Geometry check sheet. Reference: the model listing, model coordinates, mm. Face numbers are marked on the shaded views. A direction names the side the tool comes from. Coordinates: 2 decimals unless noted, no trailing zeros. Loops run counter-clockwise (first coordinate to the right, second up) from the corner with the lowest first, then second, coordinate; pieces in that order, holes last. Notation, with made-up numbers: (-3, 83.25) - (13, 83.25) arc R21 ccw to (13, 122.25) - close; hole circle Ø1 at (85, -5.5). An arc over 180 degrees is marked (long way). Write each question's results on one line, items separated by ' | '. Start each with the question number.
(1) Sectioned sample at B-B (z = 9.1). Enter the section's corners in (x, y), plus the area to 3 significant figures.
(2) Sectioned sample at A-A (y = 128.35). Enter the section's corners in (x, z), plus the area to 3 significant figures.
(3) Sectioned sample at D-D (x = -32.5). Enter the section's corners in (y, z), plus the area to 3 significant figures.
(4) Material ranges on probe 1 along Z at (x, y) = (-34, 166.05); probe 2 along Y at (x, z) = (-12, 9); probe 3 along Z at (x, y) = (-34, 167.8), recorded low to high.
(5) Access from +Z, -Z, +X, -X, +Y, -Y to the whole of each face (thin tool, end or side, straight path). Record for the marked faces 5 and 6.
(6) Mould release check, pull along Y, two halves, no side actions. Record for the marked faces 1, 2, 3 and 4: pulls with the +Y half, pulls with the -Y half, needs draft (parallel to the pull), parting line crosses it, or undercut.
(7) Go/stop test with flat-tipped pins: pin 1 Ø8 at (x, y) = (10, 164.5) entering from +Z; pin 2 Ø6.5 at (x, z) = (11, -30) entering from -Y; pin 3 Ø11 at (x, z) = (10.5, -28) entering from -Y; pin 4 Ø2.5 at (y, z) = (159.35, 9.1) entering from -X. Record where each tip stops, or that it passes through.
(8) Sectioned sample at C-C (y = 151). Enter the section's corners in (x, z).
from build123d import *

# Parameters (mm, degrees)
SKETCH003_W   = 47.3
SKETCH003_H   = 54.75
SKETCH003_R   = 11.5
SKETCH003_R_2 = 1.65
PAD001_DEPTH  = 6
SKETCH005_R   = 2.75
PAD003_DEPTH  = 5
PAD002_DEPTH  = 4
SKETCH_R      = 5.1
POCKET_DEPTH  = 2
CHAMFER_SIZE  = 1


with BuildPart() as part:
    # Sketch003 → Pad001 (new body)
    with BuildSketch(Plane.YZ):
        with Locations((-23.65, 27.375)):
            Rectangle(SKETCH003_W, SKETCH003_H)
        with Locations((-26.15, 33.6)):
            Circle(SKETCH003_R, mode=Mode.SUBTRACT)
        with Locations((-41.65, 49.1)):
            Circle(SKETCH003_R_2, mode=Mode.SUBTRACT)
        with Locations((-10.65, 49.1)):
            Circle(SKETCH003_R_2, mode=Mode.SUBTRACT)
        with Locations((-41.65, 18.1)):
            Circle(SKETCH003_R_2, mode=Mode.SUBTRACT)
        with Locations((-10.65, 18.1)):
            Circle(SKETCH003_R_2, mode=Mode.SUBTRACT)
    extrude(amount=PAD001_DEPTH)

    # Sketch005 → Pad003 (join)
    with BuildSketch(Plane.XZ):
        Polygon((-38, 40), (-28.5, 40), (-28.5, 18), (0, 18), (0, 54.75), (6, 54.75), (36, 40), (36, 0), (-38, 0), align=None)
        with Locations((-19, 10)):
            Circle(SKETCH005_R, mode=Mode.SUBTRACT)
        with Locations((26, 30)):
            Circle(SKETCH005_R, mode=Mode.SUBTRACT)
        with Locations((26, 10)):
            Circle(SKETCH005_R, mode=Mode.SUBTRACT)
    extrude(amount=PAD003_DEPTH)

    # Sketch004 → Pad002 (join)
    with BuildSketch(Plane.XY):
        Polygon((-19, 0), (-19, -5.017162), (0, -47.3), (6, -47.3), (36, -5), (36, 0), align=None)
    extrude(amount=PAD002_DEPTH)

    # Sketch → Pocket (cut)
    with BuildSketch(Plane.XZ.offset(5)):
        with Locations((-19, 10)):
            Circle(SKETCH_R)
        with Locations((26, 30)):
            Circle(SKETCH_R)
        with Locations((26, 10)):
            Circle(SKETCH_R)
    extrude(amount=-POCKET_DEPTH, mode=Mode.SUBTRACT)

    # Chamfer
    chamfer_edges = [part.edges().sort_by_distance(p)[0] for p in [
        (3, -47.3, 54.75),
        (-28.5, -2.5, 40),
        (-38, -2.5, 40),
        (-38, -2.5, 0),
    ]]
    chamfer(chamfer_edges, length=CHAMFER_SIZE)


with BuildPart() as part_1:
    # Body001082 placement: moved
    add(part.part.moved(Location((-15, 170, -40))))


solid = part_1.part
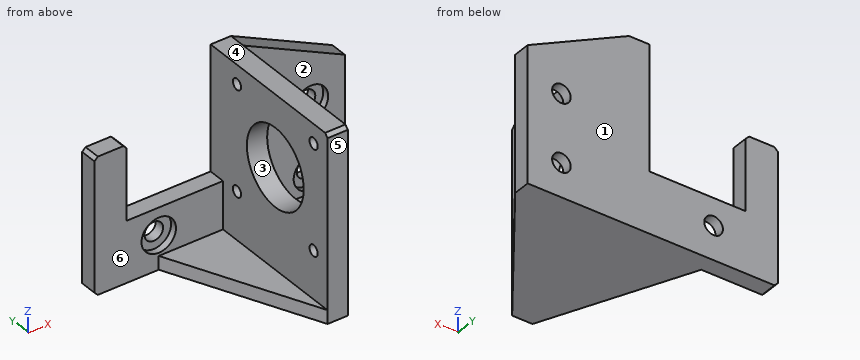
Outcome:
1) outline: (-15, 122.7) - (-9, 122.7) - (-9, 126.7) - (-15, 126.7) - close; (-15, 130) - (-9, 130) - (-9, 157.7) - (-15, 157.7) - close; (-15, 161) - (-9, 161) - (-9, 165) - (2.49, 165) - (2.49, 170) - (-15, 170) - close | area: 302 mm2
2) outline: (-17.54, -40) - (-4.99, -40) - (-4.99, -36) - (-9, -36) - (-9, -23.55) - (-15, -23.55) - (-15, -36) - (-17.54, -36) - close; (-15, -20.25) - (-9, -20.25) - (-9, 7.45) - (-15, 7.45) - close; (-15, 10.75) - (-9, 10.75) - (-9, 14.75) - (-15, 14.75) - close | area: 315 mm2
3) outline: (161.64, -40) - (170, -40) - (170, -32.3) - (167, -32.3) - (167, -34.87) - (165, -34.87) - (165, -36) - (161.64, -36) - close; (165, -25.13) - (167, -25.13) - (167, -27.7) - (170, -27.7) - (170, -22) - (165, -22) - close | area: 70.1 mm2
4) probe 1: z = -40 to -35.1, -24.9 to -22 | probe 2: y = 122.7 to 126.7, 130 to 157.7, 161 to 170 | probe 3: z = -40 to -32.75, -27.25 to -22
5) face 5: +Z, -Z, +X, -X, -Y | face 6: +Z, -X, -Y
6) face 1: pulls with the +Y half | face 2: pulls with the -Y half | face 3: undercut | face 4: needs draft
7) pin 1: stops at z = 7.36 | pin 2: stops at y = 167 | pin 3: stops at y = 165 | pin 4: passes through
8) outline: (-27.72, -40) - (11.07, -40) - (11.07, -36) - (-9, -36) - (-9, -15.41) - (-15, -15.41) - (-15, -36) - (-27.72, -36) - close; (-15, 2.61) - (-9, 2.61) - (-9, 14.75) - (-15, 14.75) - close
